```python
from build123d import *

# Parameters (mm, degrees)
F0_R     = 14.5049581744
F1_DEPTH = 84.074
F2_R     = 1.301702719
F3_DEPTH = 84.075
F4_W     = 3.6260485649
F4_H     = 8.158609271
F6_R     = 0.7971733183


with BuildPart() as f1:
    # F0 (on Top) → F1 (new body)
    with BuildSketch(Plane.XY):
        Circle(F0_R)
    extrude(amount=F1_DEPTH)

    # F2 (on face) → F3 (cut, through all)
    with BuildSketch(Plane.XY.offset(84.074)):
        with Locations((0, 6.7397234961)):
            Circle(F2_R)
        with Locations((5.8367717621, 3.3698617481)):
            Circle(F2_R)
        with Locations((5.8367717621, -3.3698617481)):
            Circle(F2_R)
        with Locations((0, -6.7397234961)):
            Circle(F2_R)
        with Locations((-5.8367717621, -3.3698617481)):
            Circle(F2_R)
        with Locations((-5.8367717621, 3.3698617481)):
            Circle(F2_R)
    extrude(amount=-F3_DEPTH, mode=Mode.SUBTRACT)

    # F4 (on Front) → F5 (revolve, cut)
    with BuildSketch(Plane.XZ):
        with Locations((10.7324868441, 81.2547430396)):
            Rectangle(F4_W, F4_H)
    revolve(axis=Axis((0, 0, 0), (0, 0, -1)), mode=Mode.SUBTRACT)

    # F6
    f6_edges = [f1.edges().sort_by_distance(p)[0] for p in [
        (-14.504958, 0, 84.074),
        (-12.545511, 0, 84.074),
    ]]
    fillet(f6_edges, radius=F6_R)


solid = f1.part
```
Verification items for the finished model (mm, model axes). A direction names the side the tool comes from. Round coordinates to 2 decimals unless told otherwise and drop trailing zeros. Write each loop counter-clockwise with the first axis right and the second up, starting at its lowest first coordinate (ties: lowest second). Pieces come first, ordered by that corner, then holes. Notation, with made-up numbers: (-33, 83) - (22, 83) arc R18 cw to (22, 114) - close; hole circle Ø10 at (45.25, 8). An arc over 180 degrees is marked (long way). Answer as a JSON object with one key per item and string values. Group by question number.
Q1. Mould release check, pull along X, two halves, no side actions. Record for faces 3 (the cylindrical face through (-1.161, -8.844, 80.673)), 4 (the cylindrical face through (-11.51, -8.83, 41.06)), 5 (the flat face through (6, -12.1, 84.074)): released by +X, released by -X, zero draft, split by the parting line, or undercut.
Q2. Section check A-A, the plane x = 0. Enter the section's corners in (y, z).
Q3. Go/stop test with flat-tipped pins: pin 1 Ø1 at (y, z) = (11.5, 51.5) entering from +X; pin 2 Ø2 at (y, z) = (-10, 42.5) entering from +X; pin 3 Ø6 at (x, z) = (4, 61.5) entering from -Y. Record where each tip stops, or that it passes through.
Q4. Section check C-C, the plane z = 65. Enter the section's corners in (x, y), plus the area to 3 significant figures.
Q5. Thickness scan on line 1 (Y direction, x = 0, z = 82.25); line 2 (Y direction, x = 6.5, z = 11.5); line 3 (Z direction, x = -12, y = -1). Record the ranges inside material, lowest first.
Q6. Section check B-B, the plane y = 0. Enter the section's corners in (x, z).
Q7. Tool access check on faces 1 (the cylindrical face through (-2.72, 12.247, 80.269)), 2 (the cylindrical face through (-6.87, 2.58, 42.63)). Record the directions out of +Z, -Z, +X, -X, +Y, -Y that give a thin tool (end or side, any length) a straight path to the whole face; none if there is none.
Found:
{
 "1": {"face 3": "undercut", "face 4": "split by the parting line", "face 5": "zero draft"},
 "2": {"outline": "(-14.5, 0) - (-8.04, 0) - (-8.04, 84.07) - (-8.92, 84.07) - (-8.92, 77.18) - (-12.55, 77.18) - (-12.55, 83.28) arc R0.8 ccw to (-13.34, 84.07) - (-13.71, 84.07) arc R0.8 ccw to (-14.5, 83.28) - close; (-5.44, 0) - (5.44, 0) - (5.44, 84.07) - (-5.44, 84.07) - close; (8.04, 0) - (14.5, 0) - (14.5, 83.28) arc R0.8 ccw to (13.71, 84.07) - (13.34, 84.07) arc R0.8 ccw to (12.55, 83.28) - (12.55, 77.18) - (8.92, 77.18) - (8.92, 84.07) - (8.04, 84.07) - close"},
 "3": {"pin 1": "stops at x = 9.45", "pin 2": "stops at x = 11.38", "pin 3": "stops at y = -14.47"},
 "4": {"outline": "circle Ø29.01 at (0, 0); hole circle Ø2.6 at (-5.84, -3.37); hole circle Ø2.6 at (-5.84, 3.37); hole circle Ø2.6 at (0, -6.74); hole circle Ø2.6 at (0, 6.74); hole circle Ø2.6 at (5.84, -3.37); hole circle Ø2.6 at (5.84, 3.37)", "area": "629 mm^2"},
 "5": {"line 1": "y = -14.5 to -12.55, -8.92 to -8.04, -5.44 to 5.44, 8.04 to 8.92, 12.55 to 14.5", "line 2": "y = -12.97 to -4.49, -2.25 to 2.25, 4.49 to 12.97", "line 3": "z = 0 to 77.18"},
 "6": {"outline": "(-14.5, 0) - (14.5, 0) - (14.5, 83.28) arc R0.8 ccw to (13.71, 84.07) - (13.34, 84.07) arc R0.8 ccw to (12.55, 83.28) - (12.55, 77.18) - (8.92, 77.18) - (8.92, 84.07) - (-8.92, 84.07) - (-8.92, 77.18) - (-12.55, 77.18) - (-12.55, 83.28) arc R0.8 ccw to (-13.34, 84.07) - (-13.71, 84.07) arc R0.8 ccw to (-14.5, 83.28) - close"},
 "7": {"face 1": "+Z", "face 2": "+Z, -Z"}
}
